```python
from build123d import *

# Parameters (mm, degrees)
F1_DEPTH = 7.5


with BuildPart() as f1:
    # F0 (on Top) → F1 (new body)
    with BuildSketch(Plane.XY):
        Polygon((-50.989201, 2), (-52.489201, 2), (-52.489201, 0), (50.010799, 0), (50.010799, 2), (48.510799, 2), (46.381295, 2), (-50.367929, 2), align=None)
        Polygon((48.510799, 2), (50.010799, 2), (50.010799, 5), (50.010799, 10), (48.510799, 10), (48.510799, 2.672095), align=None)
        Polygon((48.510799, 2.672095), (46.381295, 2), (48.510799, 2), align=None)
        Polygon((-52.489201, 5), (-52.489201, 2), (-50.989201, 2), (-50.989201, 2.994474), (-50.989201, 10), (-52.489201, 10), align=None)
        Polygon((50.010799, 10), (50.010799, 5), (51.734168, 5.8), align=None)
        Polygon((-54.21257, 5.8), (-52.489201, 5), (-52.489201, 10), align=None)
        Polygon((-50.989201, 2.994474), (-50.989201, 2), (-50.367929, 2), align=None)
    extrude(amount=F1_DEPTH)


solid = f1.part
```
Model file for the job. Use its own axes, mm. A direction names the side the tool comes from. Round coordinates to 2 decimals unless told otherwise and drop trailing zeros. Write each loop counter-clockwise with the first axis right and the second up, starting at its lowest first coordinate (ties: lowest second). Pieces come first, ordered by that corner, then holes. Notation, with made-up numbers: (-14, -36) - (23, -36) arc R9 cw to (23, -29) - close; hole circle Ø11 at (63.25, 44). An arc over 180 degrees is marked (long way). Use CSV: the item, a comma, the result in double quotes. Start each with the question number.
Item 1: Pin check, flat tips, straight feed: P1, Ø4, axis at x = -18, z = 3, coming from the +Y side; P2, Ø2, axis at y = 7, z = 3, coming from the -X side; P3, Ø4, axis at y = 2, z = 5.5, coming from the +X side. Stop position of each tip, or through.
Item 2: Drill centre lines: L1, parallel to X at y = 4.5, z = 2.25; L2, parallel to Y at x = 43, z = 6; L3, parallel to X at y = 8.5, z = 1.5. Where is each one in solid material? Low to high. Write a range as [from, to].
Item 3: Band-saw the part on A-A (y = 8.75). Write the cut outline in (x, z), and give its area (3 significant figures).
Item 4: Band-saw the part on C-C (x = -44.5). Write the cut outline in (y, z), and give its area (3 significant figures).
Item 5: Two-plate mould, pull along X, no slides. Class faces 4 (the face through (2.4, 1.7, 7.5)), 5 (the face through (-53.363, 5.406, 3.698)), 6 (the face through (47.46, 2.34, 3.7)), 7 (the face through (50.011, 2, 4)): released by +X, released by -X, zero draft, split by the parting line, or undercut.
Item 6: Tool access for faces 1 (the face through (-50.989, 6, 4)), 2 (the face through (50.86, 5.394, 3.698)), 3 (the face through (-52.489, 3, 4)): list every direction of +Z, -Z, +X, -X, +Y, -Y with a clear straight run to the whole face (end or side of a thin tool).
Item 7: Band-saw the part on B-B (z = 4). Write the cut outline in (x, y), and give its area (3 significant figures).
Checked values:
1,P1,"stops at y = 2"
1,P2,"stops at x = -54.13"
1,P3,"stops at x = 50.01"
2,L1,"x = [-52.49, -50.99], [48.51, 50.01]"
2,L2,"y = [0, 2]"
2,L3,"x = [-53.1, -50.99], [48.51, 50.63]"
3,outline,"(-53, 0) - (-50.99, 0) - (-50.99, 7.5) - (-53, 7.5) - close; (48.51, 0) - (50.52, 0) - (50.52, 7.5) - (48.51, 7.5) - close"
3,area,"30.2 mm²"
4,outline,"(0, 0) - (2, 0) - (2, 7.5) - (0, 7.5) - close"
4,area,"15.0 mm²"
5,face 4,"zero draft"
5,face 5,"released by -X"
5,face 6,"undercut"
5,face 7,"released by +X"
6,face 1,"+Z, -Z, +Y"
6,face 2,"+Z, -Z, +X, -Y"
6,face 3,"+Z, -Z, -X, -Y"
7,outline,"(-54.21, 5.8) - (-52.49, 5) - (-52.49, 0) - (50.01, 0) - (50.01, 5) - (51.73, 5.8) - (50.01, 10) - (48.51, 10) - (48.51, 2.67) - (46.38, 2) - (-50.37, 2) - (-50.99, 2.99) - (-50.99, 10) - (-52.49, 10) - close"
7,area,"239 mm²"
